from build123d import *

# Parameters (mm, degrees)
BOSS_EXTRUDE1_DEPTH = 17
SKETCH3_W           = 58
SKETCH3_H           = 2
BOSS_EXTRUDE2_DEPTH = 2
FILLET1_R           = 3
SKETCH4_W           = 56.032437302
SKETCH4_H           = 2
BOSS_EXTRUDE3_DEPTH = 0.25
FILLET2_R           = 0.5
CUT_EXTRUDE2_REACH  = 36.923
SKETCH7_R           = 2
FILLET3_R           = 0.5


with BuildPart() as part:
    # Sketch1 → Boss-Extrude1 (new body)
    with BuildSketch(Plane.XY):
        Polygon((-26.755845082, 29), (-28.016218651, 27.2), (28.016218651, 27.2), (26.755845082, 29), (26.755845082, 29.15), (29, 29.15), (29, 31.15), (-29, 31.15), (-29, 29.15), (-26.755845082, 29.15), align=None)
    extrude(amount=-BOSS_EXTRUDE1_DEPTH)

    # Sketch3 → Boss-Extrude2 (add)
    with BuildSketch(Plane(origin=(0, 0, -17), x_dir=(-1, 0, 0), z_dir=(0, 0, -1))):
        with Locations((0, 30.15)):
            Rectangle(SKETCH3_W, SKETCH3_H)
    extrude(amount=BOSS_EXTRUDE2_DEPTH)

    # Fillet1
    fillet1_edges = [part.edges().sort_by_distance(p)[0] for p in [
        (29, 30.15, -19),
        (-29, 30.15, -19),
    ]]
    fillet(fillet1_edges, radius=FILLET1_R)

    # Sketch4 → Boss-Extrude3 (add)
    with BuildSketch(Plane.XZ.offset(-27.2)):
        with Locations((0, -2.5)):
            Rectangle(SKETCH4_W, SKETCH4_H)
    extrude(amount=BOSS_EXTRUDE3_DEPTH)

    # Fillet2
    # the kernel refuses this fillet: 0.5 mm, written as the material it takes off along each edge
    with BuildSketch(Plane(origin=(-29.098750406, 26.95, -3.5), x_dir=(0, 1, 0), z_dir=(1, 0, 0)), Plane(origin=(29.098750406, 26.95, -1.5), x_dir=(0, 1, 0), z_dir=(-1, 0, 0))) as fillet2_piece_1:
        with BuildLine():
            CenterArc((0.5, 0.433012702), FILLET2_R, 180, 60)
            Line((0, 0.433012702), (-0.01, 0.433012702))
            Line((-0.01, 0.433012702), (-0.01, 0))
            Line((-0.01, 0), (0, -0.01))
            ThreePointArc((0, -0.01), (0.125, -0.01), (0.245, -0.008660254))
            Line((0.245, -0.008660254), (0.25, 0))
        make_face()
    extrude(amount=58.197500812, mode=Mode.SUBTRACT)

    # Sketch7 → Cut-Extrude2 (cut, up to next)
    with BuildSketch(Plane(origin=(0, 31.15, 0), x_dir=(1, 0, 0), z_dir=(0, 1, 0)), mode=Mode.PRIVATE) as cut_extrude2_sk1:
        with Locations(Location((14, 13, 0), (0, 0, 270))):
            Circle(SKETCH7_R)
    cut_extrude2_tool1 = extrude(cut_extrude2_sk1.sketch, amount=-CUT_EXTRUDE2_REACH, mode=Mode.PRIVATE) & part.part
    # Sketch7 → Cut-Extrude2 (cut, up to next)
    with BuildSketch(Plane(origin=(0, 31.15, 0), x_dir=(1, 0, 0), z_dir=(0, 1, 0)), mode=Mode.PRIVATE) as cut_extrude2_sk2:
        with Locations((-14, 13)):
            Circle(SKETCH7_R)
    cut_extrude2_tool2 = extrude(cut_extrude2_sk2.sketch, amount=-CUT_EXTRUDE2_REACH, mode=Mode.PRIVATE) & part.part
    add(cut_extrude2_tool1.solids().sort_by_distance((14, 31.15, -13))[0], mode=Mode.SUBTRACT)
    add(cut_extrude2_tool2.solids().sort_by_distance((-14, 31.15, -13))[0], mode=Mode.SUBTRACT)

    # Fillet3
    fillet3_edges = [part.edges().sort_by_distance(p)[0] for p in [
        (0, 31.15, -19),
        (29, 31.15, -8),
        (-29, 31.15, -8),
        (-28.121320344, 31.15, -18.121320344),
        (28.121320344, 31.15, -18.121320344),
    ]]
    fillet(fillet3_edges, radius=FILLET3_R)


solid = part.part
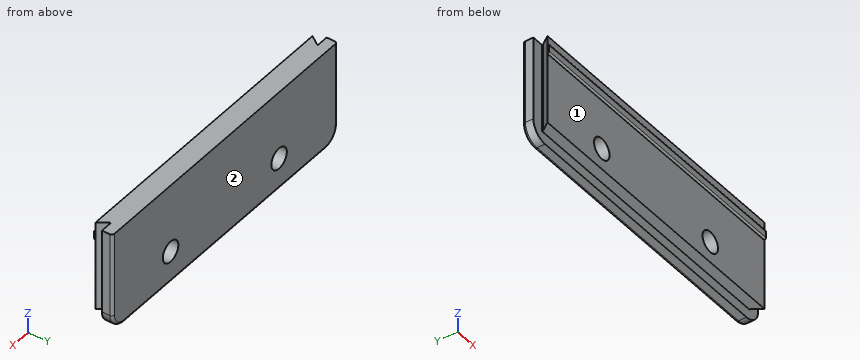
Verification items for the finished model (mm, model axes). Face numbers are marked on the shaded views. A direction names the side the tool comes from. Coordinates: 2 decimals unless noted, no trailing zeros. Loops run counter-clockwise (first coordinate to the right, second up) from the corner with the lowest first, then second, coordinate; pieces in that order, holes last. Notation, with made-up numbers: (-8, 28.5) -> (17, 28.5) arc R11 cw to (17, 47.5) -> close; hole circle Ø11 at (38.25, 70). An arc over 180 degrees is marked (long way). Answer as a JSON object with one key per item and string values. Group by question number.
Item 1: Sectioned sample at D-D on z = -6. Record the boundary of the cut face in (x, y), plus the area to 3 significant figures.
Item 2: Sectioned sample at B-B on z = -13. Record the boundary of the cut face in (x, y), plus the area to 3 significant figures.
Item 3: Scan lines: probe 1 along X at (y, z) = (30.35, -13); probe 2 along X at (y, z) = (28.8, -13); probe 3 along Y at (x, z) = (10.5, -18). Record each from-to range of solid material in increasing order.
Item 4: Depth check by flat-ended pin: pin 1 (10 mm diameter, centred on x = 8, z = -11, fed in from -Y); pin 2 (3 mm diameter, centred on x = -14, z = -13, fed in from +Y); pin 3 (1.6 mm diameter, centred on x = -6, y = 28, fed in from -Z); pin 4 (1.2 mm diameter, centred on x = 1, z = -1, fed in from -Y). Enter the tip coordinate at first touch or a pass-through.
Item 5: Sectioned sample at C-C on x = -21. Record the boundary of the cut face in (y, z), plus the area to 3 significant figures.
Item 6: Tool access check on the marked faces 1 and 2. Record the directions out of +Z, -Z, +X, -X, +Y, -Y that give a thin tool (end or side, any length) a straight path to the whole face; none if there is none.
Item 7: Sectioned sample at A-A on x = -14. Record the boundary of the cut face in (y, z), plus the area to 3 significant figures.
Evaluation:
{
 "1": {"outline": "(-29, 29.15) -> (-26.76, 29.15) -> (-26.76, 29) -> (-28.02, 27.2) -> (28.02, 27.2) -> (26.76, 29) -> (26.76, 29.15) -> (29, 29.15) -> (29, 30.65) arc R0.5 ccw to (28.5, 31.15) -> (-28.5, 31.15) arc R0.5 ccw to (-29, 30.65) -> close", "area": "223 mm²"},
 "2": {"outline": "(-29, 29.15) -> (-26.76, 29.15) -> (-26.76, 29) -> (-28.02, 27.2) -> (-16, 27.2) -> (-16, 31.15) -> (-28.5, 31.15) arc R0.5 ccw to (-29, 30.65) -> close; (-12, 27.2) -> (12, 27.2) -> (12, 31.15) -> (-12, 31.15) -> close; (16, 27.2) -> (28.02, 27.2) -> (26.76, 29) -> (26.76, 29.15) -> (29, 29.15) -> (29, 30.65) arc R0.5 ccw to (28.5, 31.15) -> (16, 31.15) -> close", "area": "191 mm²"},
 "3": {"probe 1": "x = -29 to -16, -12 to 12, 16 to 29", "probe 2": "x = -26.9 to -16, -12 to 12, 16 to 26.9", "probe 3": "y = 29.15 to 31.15"},
 "4": {"pin 1": "stops at y = 27.2", "pin 2": "passes through", "pin 3": "stops at z = -17", "pin 4": "stops at y = 27.08"},
 "5": {"outline": "(26.95, -3.07) arc R0.5 ccw to (27.2, -3.5) -> (27.2, -17) -> (29.15, -17) -> (29.15, -19) -> (30.65, -19) arc R0.5 ccw to (31.15, -18.5) -> (31.15, 0) -> (27.2, 0) -> (27.2, -1.5) arc R0.5 ccw to (26.95, -1.93) -> close", "area": "71.5 mm²"},
 "6": {"face 1": "-Z, +X, -X, -Y", "face 2": "+Z, -Z, +X, -X, +Y"},
 "7": {"outline": "(26.95, -3.07) arc R0.5 ccw to (27.2, -3.5) -> (27.2, -11) -> (31.15, -11) -> (31.15, 0) -> (27.2, 0) -> (27.2, -1.5) arc R0.5 ccw to (26.95, -1.93) -> close; (27.2, -17) -> (29.15, -17) -> (29.15, -19) -> (30.65, -19) arc R0.5 ccw to (31.15, -18.5) -> (31.15, -15) -> (27.2, -15) -> close", "area": "55.7 mm²"}
}
